Part model, mm, in its own coordinate system. A direction names the side the tool comes from. Coordinates: 2 decimals unless noted, no trailing zeros. Write each loop counter-clockwise with the first axis right and the second up, starting at its lowest first coordinate (ties: lowest second). Pieces come first, ordered by that corner, then holes. Notation, with made-up numbers: (-18.75, -21) - (27.25, -21) arc R35 cw to (27.25, 15) - close; hole circle Ø8 at (34.25, 51.25). An arc over 180 degrees is marked (long way). Write each question's results on one line, items separated by ' | '.
from build123d import *

# Parameters (mm, degrees)
SM_BASE_FLANGE_1_DEPTH = 40
CHAMFER_1_SIZE         = 5
CUT_EXTRUDE_1_DEPTH    = 206.399610516
CUT_EXTRUDE_2_DEPTH    = 204.639387153


# Sheet-metal steps are written as plain solids
with BuildPart() as part:
    # Sketch 2 → 基体-法兰1 (new, symmetric)
    with BuildSketch(Plane.XY):
        with BuildLine():
            Line((0, 190), (0, 4.5))
            ThreePointArc((0, 4.5), (-1.318019485, 1.318019485), (-4.5, 0))
            Line((-4.5, 0), (-70, 0))
            Line((-70, 0), (-70, 3))
            Line((-70, 3), (-4.5, 3))
            ThreePointArc((-4.5, 3), (-3.439339828, 3.439339828), (-3, 4.5))
            Line((-3, 4.5), (-3, 190))
            Line((-3, 190), (0, 190))
        make_face()
    extrude(amount=SM_BASE_FLANGE_1_DEPTH, both=True)

    # 倒角1
    chamfer_1_edges = [part.edges().sort_by_distance(p)[0] for p in [
        (-1.5, 190, 40),
        (-70, 1.5, 40),
        (-1.5, 190, -40),
        (-70, 1.5, -40),
    ]]
    chamfer(chamfer_1_edges, length=CHAMFER_1_SIZE)

    # 草图7 → 切除-拉伸1 (cut, through all)
    with BuildSketch(Plane.ZY.offset(3)):
        with BuildLine():
            Line((-28.9, 182), (-28.9, 152))
            ThreePointArc((-28.9, 152), (-32, 148.9), (-35.1, 152))
            Line((-35.1, 152), (-35.1, 182))
            ThreePointArc((-35.1, 182), (-32, 185.1), (-28.9, 182))
        make_face()
    cut_extrude_1 = extrude(amount=-CUT_EXTRUDE_1_DEPTH, mode=Mode.SUBTRACT)

    # 草图10 → 切除-拉伸2 (cut, through all)
    with BuildSketch(Plane(origin=(0, 3, 0), x_dir=(1, 0, 0), z_dir=(0, 1, 0))):
        with BuildLine():
            Line((-55, 34.3), (-20, 34.3))
            ThreePointArc((-20, 34.3), (-17.7, 32), (-20, 29.7))
            Line((-20, 29.7), (-55, 29.7))
            ThreePointArc((-55, 29.7), (-57.3, 32), (-55, 34.3))
        make_face()
    cut_extrude_2 = extrude(amount=-CUT_EXTRUDE_2_DEPTH, mode=Mode.SUBTRACT)

    # 镜向1: 切除-拉伸1, 切除-拉伸2 across plane
    add(cut_extrude_1.mirror(Plane.XY), mode=Mode.SUBTRACT)
    add(cut_extrude_2.mirror(Plane.XY), mode=Mode.SUBTRACT)


solid = part.part
(1) Saw through at D-D on y = 49. Write the cut outline in (x, z), then the cut area to 3 significant figures.
Return value:
outline: (-3, -40) - (0, -40) - (0, 40) - (-3, 40) - close | area: 240 mm^2
(2) 3-axis set-ups, long thin cutter, end or side, ignore diameter. For faces 1 (the flat face through (-1, 93, 40)), 2 (the flat face through (-3, 96, 1)): which of +Z, -Z, +X, -X, +Y, -Y reach the whole face in a straight line?
Return value:
face 1: +Z, +X, -X, +Y, -Y | face 2: +Z, -Z, -X, +Y
(3) Flat gauge pins, fed straight in: P1, Ø12, axis at x = -35, z = 7, coming from the +Y side; P2, Ø24, axis at y = 72.5, z = -1, coming from the -X side. Where does each tip first touch, or does it go through?
Return value:
P1: stops at y = 3 | P2: stops at x = -3
(4) Wall check: line 1 (X direction, y = 22, z = 11.5); line 2 (Y direction, x = -35, z = -16). Give the ranges that are in metal, low to high. Write a range as from..to.
Return value:
line 1: x = -3..0 | line 2: y = 0..3
(5) Saw through at B-B on z = 32. Write the cut outline in (x, y).
Return value:
outline: (-70, 0) - (-57.3, 0) - (-57.3, 3) - (-70, 3) - close; (-17.7, 0) - (-4.5, 0) arc R4.5 ccw to (0, 4.5) - (0, 148.9) - (-3, 148.9) - (-3, 4.5) arc R1.5 cw to (-4.5, 3) - (-17.7, 3) - close; (-3, 185.1) - (0, 185.1) - (0, 190) - (-3, 190) - close
(6) Saw through at A-A on x = -49. Write the cut outline in (y, z), then the cut area to 3 significant figures.
Return value:
outline: (0, -40) - (3, -40) - (3, -34.3) - (0, -34.3) - close; (0, -29.7) - (3, -29.7) - (3, 29.7) - (0, 29.7) - close; (0, 34.3) - (3, 34.3) - (3, 40) - (0, 40) - close | area: 212 mm^2
(7) Saw through at C-C on z = 11.5. Write the cut outline in (x, y), then the cut area to 3 significant figures.
Return value:
outline: (-70, 0) - (-4.5, 0) arc R4.5 ccw to (0, 4.5) - (0, 190) - (-3, 190) - (-3, 4.5) arc R1.5 cw to (-4.5, 3) - (-70, 3) - close | area: 767 mm^2
